Autodesk Inventor part; units mm, degrees
ref_plane "YZ Plane" through (0, 0, 0) normal (1, 0, 0) x (0, 1, 0)
ref_plane "XZ Plane" through (0, 0, 0) normal (0, 1, 0) x (-1, 0, 0)
ref_plane "XY Plane" through (0, 0, 0) normal (0, 0, 1) x (1, 0, 0)
sketch "スケッチ1" plane through (0, 0, 0) normal (0, 0, 1) x (1, 0, 0)
  line L0 (0, 0) -> (252.35, 0)
  line L1 (252.35, 0) -> (252.35, 70)
  line L2 (252.35, 70) -> (0, 70)
  line L3 (0, 70) -> (0, 0)
  dimension "d0" = 70
  dimension "d1" = 252.35
extrude "押し出し1" add sketch "スケッチ1" along normal blind 8
sketch "スケッチ2" plane through (0, 0, 8) normal (0, 0, 1) x (1, 0, 0)
  line L0 (0, 0) -> (252.35, 0)
  line L1 (0, 70) -> (0, 0)
  point P0 (25, 35)
  dimension "d4" = 35
  dimension "d5" = 25
hole "穴1" at (25, 35, 8) direction (0, 0, -1) diameter 24 end through all
sketch "スケッチ3" plane through (0, 0, 8) normal (0, 0, 1) x (1, 0, 0)
  line L0 (252.35, 0) -> (252.35, 70)
  circle A0 centre (25, 35) radius 12
  line L1 (0, 0) -> (252.35, 0)
  point P0 (212.35, 35)
  dimension "d14" = 187.35
  dimension "d15" = 35
hole "穴2" at (212.35, 35, 8) direction (0, 0, -1) diameter 24 end through all
sketch "スケッチ4" plane through (0, 0, 8) normal (0, 0, 1) x (1, 0, 0)
  line L0 (252.35, 0) -> (252.35, 70)
  line L1 (0, 70) -> (0, 0)
  line L2 (252.35, 70) -> (0, 70)
  line L3 (0, 0) -> (252.35, 0)
  line L4 (0, 55) -> (147.35, 55)
  line L5 (0, 15) -> (147.35, 15)
  line L6 (147.35, 0) -> (147.35, 15)
  line L7 (147.35, 55) -> (147.35, 70)
  line L8 (147.35, 55) -> (0, 55)
  line L9 (0, 55) -> (0, 70)
  line L10 (0, 70) -> (147.35, 70)
  line L11 (147.35, 70) -> (147.35, 55)
  line L12 (147.35, 15) -> (0, 15)
  line L13 (0, 15) -> (0, 0)
  line L14 (0, 0) -> (147.35, 0)
  line L15 (147.35, 0) -> (147.35, 15)
  dimension "d24" = 15
  dimension "d25" = 15
extrude "押し出し2" cut sketch "スケッチ4" against normal blind 10 contours L3 L1 L5 L6 | L7 L4 L1 L2
fillet "フィレット1" radius 4 2 edges at (147.35, 15, 4) (147.35, 55, 4)
sketch "スケッチ5" plane through (0, 0, 8) normal (0, 0, 1) x (1, 0, 0)
  line L0 (147.35, 0) -> (252.35, 0)
  circle A0 centre (212.35, 35) radius 12
  point P0 (0, 0)
  point P1 (238.35, 35)
  point P2 (199.35, 57.5167)
  point P3 (199.35, 12.4833)
  dimension "d29" = 35
  dimension "d30" = 26
  dimension "d33" = 360
hole "穴3" at (238.35, 35, 8) at (199.35, 57.5167, 8) at (199.35, 12.4833, 8) direction (0, 0, -1) diameter 3.5 end through all
sketch "スケッチ6" plane through (0, 0, 8) normal (0, 0, 1) x (1, 0, 0)
  circle A0 centre (212.35, 35) radius 12
  line L0 (147.35, 0) -> (252.35, 0)
  point P0 (0, 0)
  point P1 (194.35, 35)
  point P2 (221.35, 19.4115)
  point P3 (221.35, 50.5885)
  dimension "d42" = 18
  dimension "d43" = 35
  dimension "d46" = 360
hole "穴4" at (194.35, 35, 8) at (221.35, 19.4115, 8) at (221.35, 50.5885, 8) direction (0, 0, -1) diameter 3.5 end through all
fillet "フィレット2" radius 4 6 edges at (0, 55, 4) (0, 15, 4) (147.35, 0, 4) (147.35, 70, 4) (252.35, 70, 4) (252.35, 0, 4)
properties part number "タイヤアーム"
Work out the finished part from the listing and answer in its coordinate system (mm). A direction names the side the tool comes from. Round coordinates to 2 decimals unless told otherwise and drop trailing zeros. Order: outer loops, then holes, each group sorted by start corner. A loop starts at its lowest first (then second) coordinate and runs counter-clockwise, first axis right, second up. Notation, with made-up numbers: M 72,76.5 L 117,76.5 A27 ccw 117,95.5 Z; hole C 24.5,43.5 d2. An arc over 180 degrees is marked long. Put each result on its own line as item: value. Start each with the question number.
Q1. Section B-B, the plane z = 2 is taken. Give the number of separate pieces and of enclosed holes in the cut face, and give its area (3 significant figures).
Q2. Section A-A, the plane x = 25 is taken. Write down the section's boundary in (y, z), and give its area (3 significant figures).
Q3. Section D-D, the plane x = 76 is taken. Write down the section's boundary in (y, z).
Q4. A tool of negligible diameter and unlimited length cuts with its end or side. For faces 1 (the flat face through (152, 35, 8)), 2 (the flat face through (73, 15, 4)), 3 (the flat face through (73, 55, 4)), from which of +Z, -Z, +X, -X, +Y, -Y can it reach the whole face along a straight path? Write none if from no direction.
Q5. Flat-ended cylindrical pins translate along their axes: pin 1 (5.5 mm diameter, centred on x = 194.35, y = 35, fed in from -Z); pin 2 (1.5 mm diameter, centred on x = 84, z = 6, fed in from +Y); pin 3 (3.5 mm diameter, centred on y = 6, z = 3, fed in from -X); pin 4 (2.5 mm diameter, centred on x = 57, z = 3.5, fed in from -Y). Find the tip coordinate at first contact, or state that the pin passes through.
Q6. Straight lines are drawn through the part: L1, parallel to X at y = 35, z = 6; L2, parallel to Y at x = 199.35, z = 6; L3, parallel to X at y = 42.5, z = 1. For each, find the intervals that lie inside material, in ascending order. Write a range as [from, to].
Q7. For a pull along X with two mould halves and no side action, classify faces 4 (the flat face through (0, 35, 4)), 5 (the cylindrical face through (224.065, 37.601, 3.944)), 6 (the flat face through (152, 35, 0)) as pulls with the +X half, pulls with the -X half, needs draft (parallel to the pull), parting line crosses it, or undercut.
Q8. Section C-C, the plane y = 7.5 is taken. Write down the section's boundary in (x, z), and give its area (3 significant figures).
Findings below:
1. separate pieces: 1
1. enclosed holes: 8
1. area: 12,300 mm^2
2. outline: M 15,0 L 23,0 L 23,8 L 15,8 Z; M 47,0 L 55,0 L 55,8 L 47,8 Z
2. area: 128 mm^2
3. outline: M 15,0 L 55,0 L 55,8 L 15,8 Z
4. face 1: +Z, +X, -X, +Y, -Y
4. face 2: +Z, -Z, -X, -Y
4. face 3: +Z, -Z, -X, +Y
5. pin 1: stops at z = 0
5. pin 2: stops at y = 55
5. pin 3: stops at x = 147.35
5. pin 4: stops at y = 15
6. L1: x = [0, 13], [37, 192.6], [196.1, 200.35], [224.35, 236.6], [240.1, 252.35]
6. L2: y = [0, 10.73], [14.23, 55.77], [59.27, 70]
6. L3: x = [0, 15.63], [34.37, 202.98], [221.72, 252.35]
7. face 4: pulls with the -X half
7. face 5: undercut
7. face 6: needs draft
8. outline: M 147.35,0 L 252.35,0 L 252.35,8 L 147.35,8 Z
8. area: 840 mm^2
